```python
from build123d import *

# Parameters (mm, degrees)
BOSS_EXTRUDE1_DEPTH = 0.2
SKETCH2_R           = 0.323929716
SKETCH2_R_2         = 0.2
SKETCH2_R_3         = 0.203589937
SKETCH2_R_4         = 0.5
CUT_EXTRUDE1_DEPTH  = 1.2


with BuildPart() as part:
    # Sketch1 → Boss-Extrude1 (new body)
    with BuildSketch(Plane.XY):
        with BuildLine():
            Line((-2.296100594, 9.872845996), (-5.357568053, 8.604744654))
            ThreePointArc((-5.357568053, 8.604744654), (-7.304108146, 7.304108146), (-8.604744654, 5.357568053))
            Line((-8.604744654, 5.357568053), (-9.872845996, 2.296100594))
            ThreePointArc((-9.872845996, 2.296100594), (-10.329568801, 0), (-9.872845996, -2.296100594))
            Line((-9.872845996, -2.296100594), (-8.604744654, -5.357568053))
            ThreePointArc((-8.604744654, -5.357568053), (-7.304108146, -7.304108146), (-5.357568053, -8.604744654))
            Line((-5.357568053, -8.604744654), (-2.296100594, -9.872845996))
            ThreePointArc((-2.296100594, -9.872845996), (0, -10.329568801), (2.296100594, -9.872845996))
            Line((2.296100594, -9.872845996), (5.357568053, -8.604744654))
            ThreePointArc((5.357568053, -8.604744654), (7.304108146, -7.304108146), (8.604744654, -5.357568053))
            Line((8.604744654, -5.357568053), (9.872845996, -2.296100594))
            ThreePointArc((9.872845996, -2.296100594), (10.329568801, 0), (9.872845996, 2.296100594))
            Line((9.872845996, 2.296100594), (8.604744654, 5.357568053))
            ThreePointArc((8.604744654, 5.357568053), (7.304108146, 7.304108146), (5.357568053, 8.604744654))
            Line((5.357568053, 8.604744654), (2.296100594, 9.872845996))
            ThreePointArc((2.296100594, 9.872845996), (0, 10.329568801), (-2.296100594, 9.872845996))
        make_face()
    extrude(amount=BOSS_EXTRUDE1_DEPTH)

    # Sketch2 → Cut-Extrude1 (cut, through all)
    with BuildSketch(Plane(origin=(0, 0, 0), x_dir=(-1, 0, 0), z_dir=(0, 0, -1))):
        with Locations((0, -6.5)):
            Circle(SKETCH2_R)
        with Locations((-4, -5.25)):
            Circle(SKETCH2_R_2)
        with Locations((4, -5.25)):
            Circle(SKETCH2_R_3)
        with Locations((4, 5.25)):
            Circle(SKETCH2_R_2)
        with Locations((0, 6.5)):
            Circle(SKETCH2_R)
        with Locations((-4, 5.25)):
            Circle(SKETCH2_R_2)
        with Locations((4, 0)):
            Circle(SKETCH2_R_4)
        with Locations((-4, 0)):
            Circle(SKETCH2_R_4)
    extrude(amount=-CUT_EXTRUDE1_DEPTH, mode=Mode.SUBTRACT)


solid = part.part
```
CAD build for the part. Positions are in the model's coordinates, mm. Round coordinates to 2 decimals unless told otherwise and drop trailing zeros. Loops run counter-clockwise (first coordinate to the right, second up) from the corner with the lowest first, then second, coordinate; pieces in that order, holes last. Notation, with made-up numbers: M 77,40 L 101,40 A18 ccw 101,75 Z; hole C 89.25,4.5 d1. An arc over 180 degrees is marked long. Return JSON: item names as keys, results as strings. Group by question number.
(1) Saw through at B-B, the plane z = 0.1. Give the number of separate pieces and of enclosed holes in the cut face, and give its area (3 significant figures).
(2) Saw through at C-C, the plane y = 6.5. List the corners of the cut face in (x, z).
(3) Saw through at A-A, the plane x = 0. List the corners of the cut face in (y, z).
(4) Wall check: probe 1 along Y at (x, z) = (0, 0.15); probe 2 along Y at (x, z) = (0.25, 0.15); probe 3 along Y at (x, z) = (-4, 0.1). Give the ranges that are in metal, low to high. Write a range as [from, to].
(5) Saw through at D-D, the plane y = -4. List the corners of the cut face in (x, z), and give its area (3 significant figures).
Answer list:
{
 "1": {"separate pieces": "1", "enclosed holes": "8", "area": "322 mm2"},
 "2": {"outline": "M -7.98,0 L -0.32,0 L -0.32,0.2 L -7.98,0.2 Z; M 0.32,0 L 7.98,0 L 7.98,0.2 L 0.32,0.2 Z"},
 "3": {"outline": "M -10.33,0 L -6.82,0 L -6.82,0.2 L -10.33,0.2 Z; M -6.18,0 L 6.18,0 L 6.18,0.2 L -6.18,0.2 Z; M 6.82,0 L 10.33,0 L 10.33,0.2 L 6.82,0.2 Z"},
 "4": {"probe 1": "[-10.33, -6.82], [-6.18, 6.18], [6.82, 10.33]", "probe 2": "[-10.32, -6.71], [-6.29, 6.29], [6.71, 10.32]", "probe 3": "[-9.17, -5.45], [-5.05, -0.5], [0.5, 5.05], [5.45, 9.17]"},
 "5": {"outline": "M -9.17,0 L 9.17,0 L 9.17,0.2 L -9.17,0.2 Z", "area": "3.67 mm2"}
}
